```python
from build123d import *

# Parameters (mm, degrees)
F0_W     = 107.95
F0_H     = 107.95
F0_W_2   = 9.32
F0_H_2   = 14.5
F0_R     = 1.5
F0_H_3   = 30.63
F1_DEPTH = 5
F2_DEPTH = 3
F3_DEPTH = 5
F4_R     = 1


with BuildPart() as f1:
    # F0 (on Top) → F1 (new body)
    with BuildSketch(Plane.XY):
        with Locations((0, 36.13)):
            Rectangle(F0_W, F0_H)
        Polygon((6.16, 42.13), (6.16, 10), (6.16, -6), (0, -6), (-6.16, -6), (-6.16, 10), (-6.16, 42.13), (0, 42.13), align=None, mode=Mode.SUBTRACT)
        Polygon((6.16, 10), (4.66, 10), (4.66, -4.5), (-4.66, -4.5), (-4.66, 10), (-6.16, 10), (-6.16, -6), (0, -6), (6.16, -6), align=None)
        with Locations((0, 2.75)):
            Rectangle(F0_W_2, F0_H_2)
        Circle(F0_R, mode=Mode.SUBTRACT)
        with Locations((0, 7)):
            Circle(F0_R, mode=Mode.SUBTRACT)
        with Locations((0, 25.315)):
            Rectangle(F0_W_2, F0_H_3)
        with Locations((0, 29.13)):
            Circle(F0_R, mode=Mode.SUBTRACT)
        with Locations((0, 36.13)):
            Circle(F0_R, mode=Mode.SUBTRACT)
        Polygon((-4.66, 40.63), (4.66, 40.63), (4.66, 10), (6.16, 10), (6.16, 42.13), (0, 42.13), (-6.16, 42.13), (-6.16, 10), (-4.66, 10), align=None)
        with Locations((0, 29.13)):
            Circle(F0_R)
        with Locations((0, 36.13)):
            Circle(F0_R)
        with Locations((0, 7)):
            Circle(F0_R)
        Circle(F0_R)
    extrude(amount=F1_DEPTH)

    # F0 (on Top) → F2 (cut)
    with BuildSketch(Plane.XY):
        Polygon((-4.66, 40.63), (4.66, 40.63), (4.66, 10), (6.16, 10), (6.16, 42.13), (0, 42.13), (-6.16, 42.13), (-6.16, 10), (-4.66, 10), align=None)
        with Locations((0, 25.315)):
            Rectangle(F0_W_2, F0_H_3)
        with Locations((0, 29.13)):
            Circle(F0_R, mode=Mode.SUBTRACT)
        with Locations((0, 36.13)):
            Circle(F0_R, mode=Mode.SUBTRACT)
        with Locations((0, 29.13)):
            Circle(F0_R)
        with Locations((0, 36.13)):
            Circle(F0_R)
    extrude(amount=F2_DEPTH, mode=Mode.SUBTRACT)

    # F0 (on Top) → F3 (cut, through all)
    with BuildSketch(Plane.XY):
        Circle(F0_R)
        with Locations((0, 7)):
            Circle(F0_R)
    extrude(amount=F3_DEPTH, mode=Mode.SUBTRACT)

    # F4
    f4_edges = [f1.edges().sort_by_distance(p)[0] for p in [
        (6.16, 42.13, 1.5),
        (6.16, 10, 1.5),
        (-53.975, 90.105, 2.5),
        (53.975, 90.105, 2.5),
        (-53.975, -17.845, 2.5),
        (-6.16, 42.13, 1.5),
        (53.975, -17.845, 2.5),
        (-6.16, 10, 1.5),
        (-1.5, 7, 0),
        (-1.5, 0, 0),
        (-1.5, 7, 5),
        (-1.5, 0, 5),
    ]]
    fillet(f4_edges, radius=F4_R)


solid = f1.part
```
Build history of the part. All positions in model axes, mm. A direction names the side the tool comes from. Give positions to 0.01 mm unless a question says otherwise; leave off trailing zeros. Loops run counter-clockwise (first coordinate to the right, second up) from the corner with the lowest first, then second, coordinate; pieces in that order, holes last.
Item 1: Slice it at A-A, the plane x = 0. List the corners of the cut face in (y, z) (3 decimals), and give its area (3 significant figures).
Answers follow:
outline: (-17.845, 0) - (-2.5, 0) arc R1 ccw to (-1.5, 1) - (-1.5, 4) arc R1 ccw to (-2.5, 5) - (-17.845, 5) - close; (1.5, 1) arc R1 ccw to (2.5, 0) - (4.5, 0) arc R1 ccw to (5.5, 1) - (5.5, 4) arc R1 ccw to (4.5, 5) - (2.5, 5) arc R1 ccw to (1.5, 4) - close; (8.5, 1) arc R1 ccw to (9.5, 0) - (10, 0) - (10, 3) - (42.13, 3) - (42.13, 0) - (90.105, 0) - (90.105, 5) - (9.5, 5) arc R1 ccw to (8.5, 4) - close
area: 412 mm2
Item 2: Slice it at C-C, the plane y = 14.5. List the corners of the cut face in (x, z) (3 decimals).
Answers follow:
outline: (-53.975, 0) - (-6.16, 0) - (-6.16, 3) - (6.16, 3) - (6.16, 0) - (53.975, 0) - (53.975, 5) - (-53.975, 5) - close
Item 3: Slice it at B-B, the plane y = 0. List the corners of the cut face in (x, z) (3 decimals).
Answers follow:
outline: (-53.975, 0) - (-2.5, 0) arc R1 ccw to (-1.5, 1) - (-1.5, 4) arc R1 ccw to (-2.5, 5) - (-53.975, 5) - close; (1.5, 1) arc R1 ccw to (2.5, 0) - (53.975, 0) - (53.975, 5) - (2.5, 5) arc R1 ccw to (1.5, 4) - close
Item 4: Drill centre lines: line 1 (Y direction, x = 0, z = 1.6) (3 decimals); line 2 (Y direction, x = 0, z = 3.25) (3 decimals); line 3 (X direction, y = 27, z = 2.45) (3 decimals). Where is each one in solid material? Low to high.
Answers follow:
line 1: y = -17.845 to -1.5, 1.5 to 5.5, 8.5 to 10, 42.13 to 90.105
line 2: y = -17.845 to -1.5, 1.5 to 5.5, 8.5 to 90.105
line 3: x = -53.975 to -6.16, 6.16 to 53.975
Item 5: Pull direction Y, two halves, no side cores. Call faces 1 (the face through (-1, -17.845, 2)), 2 (the face through (-1.5, 0.07, 2.48)), 3 (the face through (0, 42.13, 1)), 4 (the face through (-53.975, 35, 2)): released by +Y, released by -Y, zero draft, split by the parting line, or undercut.
Answers follow:
face 1: released by -Y
face 2: undercut
face 3: undercut
face 4: zero draft
Item 6: Flat gauge pins, fed straight in: pin 1 (6 mm diameter, centred on x = 2.5, y = 28.5, fed in from -Z); pin 2 (4 mm diameter, centred on x = 0, y = 7, fed in from +Z); pin 3 (2.5 mm diameter, centred on x = 0, y = 0, fed in from -Z). Where does each tip first touch, or does it go through?
Answers follow:
pin 1: stops at z = 3
pin 2: stops at z = 4.87
pin 3: passes through
Item 7: Which spindle directions (+Z, -Z, +X, -X, +Y, -Y) get a long thin tool onto all of the face, cutting with end or side? Do faces 5 (the face through (0, 26, 3)), 6 (the face through (-1, 90.105, 2)). Say none if no direction does.
Answers follow:
face 5: -Z
face 6: +Z, -Z, +X, -X, +Y
